Geometry: final body of the model. Coordinates: model frame, mm. A direction names the side the tool comes from. Give positions to 0.01 mm unless a question says otherwise; leave off trailing zeros. Write each loop counter-clockwise with the first axis right and the second up, starting at its lowest first coordinate (ties: lowest second). Pieces come first, ordered by that corner, then holes. Notation, with made-up numbers: M 2,18 L 25,18 A32 cw 25,45 Z; hole C 18.5,60.25 d7. An arc over 180 degrees is marked long. Use one line per item in the form item = value. Start each with the question number.
Item 1: Section query B-B on x = 940. Give the number of separate pieces and of enclosed holes in the cut face, then the cut area to 3 significant figures.
Item 2: Section query D-D on z = 210. Return loops of the section in (x, y), then the cut area to 3 significant figures.
Item 3: Contact query for flat-ended pins moving along their axis: P1, Ø2.5, axis at x = 2494, z = 264.5, coming from the -Y side; P2, Ø10, axis at x = 1731.5, z = 196, coming from the +Y side; P3, Ø4, axis at x = 1207.5, z = 93, coming from the +Y side. Output: stop coordinate, or through.
Item 4: Material intervals for line 1 along X through (y, z) = (790, 101); line 2 along Y through (x, z) = (137.5, 329); line 3 along Y through (x, z) = (1936, 199), sorted ascending. Write a range as from..to.
Item 5: Section query A-A on y = 665. Return loops of the section in (x, z), then the cut area to 3 significant figures.
Item 6: Pull-direction query (X, two-part tool) for faces 1 (the flat face through (1612, 359, 8)), 2 (the flat face through (1415, 858, 8)), 3 (the flat face through (710, 674, 396)), 4 (the flat face through (1617, 756, 259)); classes: released by +X, released by -X, zero draft, split by the parting line, or undercut.
Item 7: Section query C-C on y = 323.5. Return loops of the section in (x, z), then the cut area to 3 significant figures.
Item 8: Access query for faces 5 (the flat face through (720, 723, 391)), 6 (the flat face through (2190, 778, 132)), 7 (the flat face through (1612, 651, 0)), 8 (the flat face through (1300, 137, 255)), 9 (the flat face through (975, 145, 391)). Directions: +Z, -Z, +X, -X, +Y, -Y. A direction counts if a zero-diameter tool reaches every point of the face in a straight line with its end or side. Return the directions, or none.
from build123d import *

# Parameters (mm, degrees)
EXTRUDE_1_DEPTH  = 8
EXTRUDE_2_DEPTH  = 8
EXTRUDE_3_DEPTH  = 8
SKETCH_7_W       = 1830
SKETCH_7_H       = 637
EXTRUDE_4_DEPTH  = 8
EXTRUDE_5_DEPTH  = 251
EXTRUDE_6_DEPTH  = 251
SKETCH_13_W      = 710
SKETCH_13_H      = 251
EXTRUDE_7_DEPTH  = 13
EXTRUDE_8_DEPTH  = 10
EXTRUDE_9_DEPTH  = 10
EXTRUDE_10_DEPTH = 1120
EXTRUDE_11_DEPTH = 1120


with BuildPart() as part:
    # ｽｹｯﾁ2 → ﾎﾞｽ - 押し出し1 (new body)
    with BuildSketch(Plane.XY.offset(259)):
        Polygon((0, 145), (2540, 145), (2540, 778), (1830, 778), (1830, 961), (710, 961), (710, 778), (0, 778), align=None)
    extrude(amount=EXTRUDE_1_DEPTH)

    # ｽｹｯﾁ4 → ﾎﾞｽ - 押し出し2 (add)
    with BuildSketch(Plane(origin=(0, 137, 0), x_dir=(1, 0, 0), z_dir=(0, 1, 0))):
        Polygon((95, -259), (710, -259), (710, -8), (2445, -8), (2445, -267), (1830, -267), (1830, -518), (95, -518), align=None)
    extrude(amount=EXTRUDE_2_DEPTH)

    # ｽｹｯﾁ5 → ﾎﾞｽ - 押し出し3 (add)
    with BuildSketch(Plane.XY):
        Polygon((710, 137), (2540, 137), (2540, 778), (1830, 778), (1830, 1150), (710, 1150), align=None)
    extrude(amount=EXTRUDE_3_DEPTH)

    # ｽｹｯﾁ7 → ﾎﾞｽ - 押し出し4 (add)
    with BuildSketch(Plane.XY.offset(518)):
        with Locations((915, 445.5)):
            Rectangle(SKETCH_7_W, SKETCH_7_H)
    extrude(amount=EXTRUDE_4_DEPTH)

    # ｽｹｯﾁ9 → ﾎﾞｽ - 押し出し5 (add)
    with BuildSketch(Plane.XY.offset(8)):
        Polygon((710, 574.32489), (2540, 548.7543), (2540, 556.7543), (710, 582.32489), align=None)
    extrude(amount=EXTRUDE_5_DEPTH)

    # ｽｹｯﾁ11 → ﾎﾞｽ - 押し出し6 (add)
    with BuildSketch(Plane.XY.offset(267)):
        Polygon((0, 548.7543), (1830, 574.32489), (1830, 582.32489), (0, 556.7543), align=None)
    extrude(amount=EXTRUDE_6_DEPTH)

    # ｽｹｯﾁ13 → ﾎﾞｽ - 押し出し7 (add)
    with BuildSketch(Plane(origin=(0, 765, 0), x_dir=(1, 0, 0), z_dir=(0, 1, 0))):
        with Locations((355, -392.5)):
            Rectangle(SKETCH_13_W, SKETCH_13_H)
        with Locations((2185, -133.5)):
            Rectangle(SKETCH_13_W, SKETCH_13_H)
    extrude(amount=EXTRUDE_7_DEPTH)

    # ｽｹｯﾁ15 → ﾎﾞｽ - 押し出し8 (add)
    with BuildSketch(Plane(origin=(710, 0, 0), x_dir=(0, 0, -1), z_dir=(1, 0, 0))):
        Polygon((-8, 572), (-259, 572), (-259, 961.319833243), (-8, 1150.461899818), align=None)
        Polygon((-267, 572), (-518, 572), (-518, 763.64506295), (-267, 952.787129526), align=None)
    extrude(amount=EXTRUDE_8_DEPTH)

    # ｽｹｯﾁ17 → ﾎﾞｽ - 押し出し9 (add)
    with BuildSketch(Plane(origin=(1820, 0, 0), x_dir=(0, 0, -1), z_dir=(1, 0, 0))):
        Polygon((-8, 572), (-259, 572), (-259, 961.319833243), (-8, 1150.461899818), align=None)
        Polygon((-267, 572), (-518, 572), (-518, 763.64506295), (-267, 952.787129526), align=None)
    extrude(amount=EXTRUDE_9_DEPTH)

    # ｽｹｯﾁ18 → ﾎﾞｽ - 押し出し10 (add)
    with BuildSketch(Plane(origin=(710, 0, 0), x_dir=(0, 0, -1), z_dir=(1, 0, 0))):
        Polygon((-12.14, 1154.855), (-262.14, 966.466487474), (-258.529109861, 961.674674414), (-8.529109861, 1150.06318694), align=None)
    extrude(amount=EXTRUDE_10_DEPTH)

    # ｽｹｯﾁ19 → ﾎﾞｽ - 押し出し11 (add)
    with BuildSketch(Plane(origin=(710, 0, 0), x_dir=(0, 0, -1), z_dir=(1, 0, 0))):
        Polygon((-272.34, 958.780236163), (-522.34, 770.391723638), (-517.525479815, 764.002639557), (-267.525479815, 952.391152083), align=None)
    extrude(amount=EXTRUDE_11_DEPTH)


solid = part.part
Answer sheet:
q1.separate_pieces = 3
q1.enclosed_holes = 2
q1.area = 32,200 mm2
q2.outline = M 710,137 L 2445,137 L 2445,145 L 710,145 Z; M 710,572 L 720,572 L 720,574.19 L 2540,548.75 L 2540,556.75 L 720,582.19 L 720,998.24 L 1820,998.24 L 1820,572 L 1830,572 L 1830,765 L 2540,765 L 2540,778 L 1830,778 L 1830,1005.76 L 710,1005.76 Z
q2.area = 54,600 mm2
q3.P1 = 145
q3.P2 = 1020.07
q3.P3 = 1095.43
q4.line_1 = 710..720, 1820..1830
q4.line_2 = 137..145, 550.68..558.68, 765..778
q4.line_3 = 137..145, 557.19..565.19, 765..778
q5.outline = M 0,259 L 710,259 L 710,0 L 2540,0 L 2540,8 L 1830,8 L 1830,259 L 2540,259 L 2540,267 L 1830,267 L 1830,526 L 0,526 L 0,518 L 710,518 L 710,267 L 0,267 Z; hole M 720,8 L 1820,8 L 1820,259 L 720,259 Z; hole M 720,267 L 1820,267 L 1820,518 L 720,518 Z
q5.area = 59,600 mm2
q6.face_1 = zero draft
q6.face_2 = undercut
q6.face_3 = released by -X
q6.face_4 = undercut
q7.outline = M 0,259 L 2540,259 L 2540,267 L 0,267 Z; M 0,518 L 1830,518 L 1830,526 L 0,526 Z; M 710,0 L 2540,0 L 2540,8 L 710,8 Z
q7.area = 49,600 mm2
q8.face_5 = none
q8.face_6 = +Z, -Z, +X, +Y
q8.face_7 = -Z, +X, -X, +Y, -Y
q8.face_8 = -Z, +X, -X, -Y
q8.face_9 = +X, -X
